```python
from build123d import *

# Parameters (mm, degrees)
F3_D          = 6
F3_DEPTH      = 20
F3_TIP        = 1.8025818571
F4_R          = 1
F5_DEPTH      = 8.001
F5_DEPTH_BACK = 8.001


with BuildPart() as f1:
    # F0 (on Front) → F1 (revolve)
    with BuildSketch(Plane.XZ):
        with BuildLine():
            Line((-8, 0), (-1.5, 0))
            Line((-1.5, 0), (-1.5, 145))
            Line((-1.5, 145), (0, 145))
            Line((0, 145), (0, 150))
            ThreePointArc((0, 150), (-2.0861816349, 149.1565641032), (-3, 147.100238759))
            Line((-3, 147.100238759), (-8, 0))
        make_face()
    revolve(axis=Axis((0, 0, -15.0155443698), (0, 0, -1)))

    # F3
    with Locations(Plane(origin=(0, 0, 0), x_dir=(1, 0, 0), z_dir=(0, 0, -1))):
        with Locations((0, 0)):
            Hole(F3_D / 2, depth=F3_DEPTH)
            with Locations((0, 0, -(F3_DEPTH + F3_TIP / 2))):  # 118° drill point
                Cone(0, F3_D / 2, F3_TIP, mode=Mode.SUBTRACT)

    # F4 (on Front) → F5 (cut, two sides)
    with BuildSketch(Plane.XZ) as f5_sk:
        with Locations((0, 145)):
            Circle(F4_R)
    extrude(amount=-F5_DEPTH, mode=Mode.SUBTRACT)
    extrude(f5_sk.sketch, amount=F5_DEPTH_BACK, mode=Mode.SUBTRACT)


solid = f1.part
```
Build history of the part. All positions in model axes, mm. Round coordinates to 2 decimals unless told otherwise and drop trailing zeros. Loops run counter-clockwise (first coordinate to the right, second up) from the corner with the lowest first, then second, coordinate; pieces in that order, holes last.
Item 1: Drill centre lines: line 1 along X through (y, z) = (0, 62); line 2 along X through (y, z) = (1.7, 145); line 3 along Y through (x, z) = (0, 99.5). Where is each one in solid material? Low to high.
Item 2: Two-plate mould, pull along X, no slides. Class faces 1 (the face through (3, 0, 10)), 2 (the face through (-3.4, 0.1, 0)), 3 (the face through (1.2, -5.403, 72.52)): released by +X, released by -X, zero draft, split by the parting line, or undercut.
Item 3: Pin check, flat tips, straight feed: P1, Ø4, axis at x = 0, y = 0, coming from the -Z side; P2, Ø3, axis at y = -3.5, z = 76, coming from the +X side; P3, Ø1.5, axis at x = 2, z = 56, coming from the -Y side. Stop position of each tip, or through.
Item 4: Saw through at A-A (z = 82). List the corners of the cut face in (x, y), then the cut area to 3 significant figures.
Item 5: Saw through at B-B (z = 50.5). List the corners of the cut face in (x, y), then the cut area to 3 significant figures.
Worked answers:
1. line 1: x = -5.89 to -1.5, 1.5 to 5.89
1. line 2: x = -2.56 to -1, 1 to 2.56
1. line 3: y = -4.62 to -1.5, 1.5 to 4.62
2. face 1: undercut
2. face 2: zero draft
2. face 3: split by the parting line
3. P1: stops at z = 20.6
3. P2: stops at x = 5.04
3. P3: stops at y = -5.97
4. outline: circle Ø10.43 at (0, 0); hole circle Ø3 at (0, 0)
4. area: 78.3 mm2
5. outline: circle Ø12.57 at (0, 0); hole circle Ø3 at (0, 0)
5. area: 117 mm2
